CAD build for the part. Positions are in the model's coordinates, mm. Face numbers are marked on the shaded views. A direction names the side the tool comes from. Coordinates: 2 decimals unless noted, no trailing zeros. Write each loop counter-clockwise with the first axis right and the second up, starting at its lowest first coordinate (ties: lowest second). Pieces come first, ordered by that corner, then holes.
```python
from build123d import *

# Parameters (mm, degrees)
SKETCH_1_W          = 40
SKETCH_1_H          = 40
EXTRUDE_1_DEPTH     = 10
SKETCH_2_W          = 10
SKETCH_2_H          = 23
EXTRUDE_2_DEPTH     = 16
SKETCH_3_R          = 1.5
CUT_EXTRUDE_1_DEPTH = 30
FILLET_2_R          = 5


with BuildPart() as part:
    # 草图1 → 凸台-拉伸1 (new body)
    with BuildSketch(Plane.XY):
        Rectangle(SKETCH_1_W, SKETCH_1_H)
    extrude(amount=EXTRUDE_1_DEPTH)

    # 草图2 → 凸台-拉伸2 (add)
    with BuildSketch(Plane.ZY.offset(20)):
        with Locations((5, 0)):
            Rectangle(SKETCH_2_W, SKETCH_2_H)
    extrude_2 = extrude(amount=EXTRUDE_2_DEPTH)

    # 草图3 → 切除-拉伸1 (cut)
    with BuildSketch(Plane(origin=(0, 11.5, 0), x_dir=(1, 0, 0), z_dir=(0, 1, 0))):
        with Locations(Location((-30, -5, 0), (0, 0, 180))):
            Circle(SKETCH_3_R)
    cut_extrude_1 = extrude(amount=-CUT_EXTRUDE_1_DEPTH, mode=Mode.SUBTRACT)

    # 镜向1: 凸台-拉伸2, 切除-拉伸1 across plane
    add(extrude_2.mirror(Plane(origin=(0, 0, 0), x_dir=(0, 0, 1), z_dir=(1, 0, 0))))
    add(cut_extrude_1.mirror(Plane(origin=(0, 0, 0), x_dir=(0, 0, 1), z_dir=(1, 0, 0))), mode=Mode.SUBTRACT)

    # 圆角2
    fillet_2_edges = [part.edges().sort_by_distance(p)[0] for p in [
        (36, 0, 0),
        (36, 0, 10),
    ]]
    fillet(fillet_2_edges, radius=FILLET_2_R - 0.0001)  # a hair under: the kernel refuses the full size


solid = part.part
```
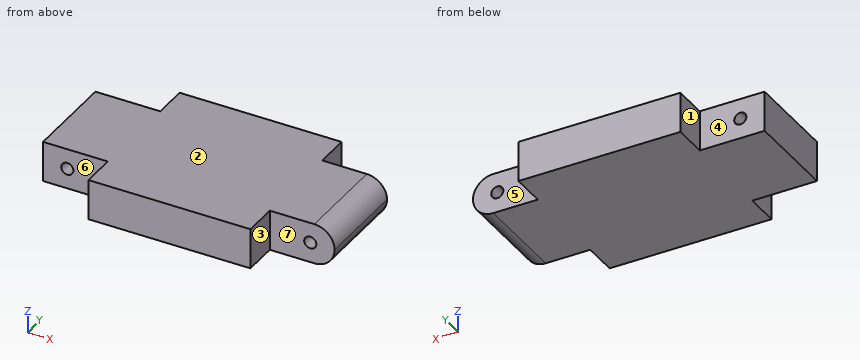
Item 1: Saw through at D-D, the plane x = 23.5. Write the cut outline in (y, z).
Item 2: Which spindle directions (+Z, -Z, +X, -X, +Y, -Y) get a long thin tool onto all of the face, cutting with end or side? Do the marked faces 4, 5, 6 and 7. Say none if no direction does.
Item 3: Flat gauge pins, fed straight in: pin 1 Ø3 at (x, z) = (26.5, 5.5) entering from +Y; pin 2 Ø3 at (x, z) = (31.5, 5) entering from -Y; pin 3 Ø4 at (x, y) = (-26.5, 10.5) entering from -Z. Where does each tip first touch, or does it go through?
Item 4: Two-plate mould, pull along X, no slides. Class the marked faces 1, 2 and 3: +X half, -X half, draft (parallel to the pull), parting line (faces both ways), or undercut.
Item 5: Saw through at A-A, the plane x = -30. Write the cut outline in (y, z).
Item 6: Saw through at B-B, the plane y = -10. State how many separate pieces and enclosed holes the cut face has, and give its area (3 significant figures).
Item 7: Wall check: line 1 along X through (y, z) = (-11, 6); line 2 along Z through (x, y) = (30, 4.5); line 3 along X through (y, z) = (-1.5, 4.5). Give the ranges that are in metal, low to high.
Item 8: Saw through at C-C, the plane z = 8.75. Write the cut outline in (x, y), and give its area (3 significant figures).
Working result:
1. outline: (-11.5, 0) - (11.5, 0) - (11.5, 10) - (-11.5, 10) - close
2. face 4: +Z, -Z, -X, +Y
2. face 5: +Z, -Z, +X, +Y
2. face 6: +Z, -Z, -X, -Y
2. face 7: +Z, -Z, +X, -Y
3. pin 1: stops at y = 11.5
3. pin 2: stops at y = -11.5
3. pin 3: stops at z = 0
4. face 1: -X half
4. face 2: draft
4. face 3: +X half
5. outline: (-11.5, 0) - (11.5, 0) - (11.5, 3.5) - (-11.5, 3.5) - close; (-11.5, 6.5) - (11.5, 6.5) - (11.5, 10) - (-11.5, 10) - close
6. separate pieces: 1
6. enclosed holes: 2
6. area: 695 mm2
7. line 1: x = -36 to -31.12, -28.88 to 28.88, 31.12 to 35.9
7. line 2: z = 0 to 3.5, 6.5 to 10
7. line 3: x = -36 to -31.41, -28.59 to 28.59, 31.41 to 35.97
8. outline: (-36, -11.5) - (-20, -11.5) - (-20, -20) - (20, -20) - (20, -11.5) - (34.31, -11.5) - (34.31, 11.5) - (20, 11.5) - (20, 20) - (-20, 20) - (-20, 11.5) - (-36, 11.5) - close
8. area: 2,300 mm2
